Check sheet for the modelled part. Datum: model origin and axes. Units: mm. Face numbers are marked on the shaded views. A direction names the side the tool comes from. Round coordinates to 2 decimals unless told otherwise and drop trailing zeros. Write each loop counter-clockwise with the first axis right and the second up, starting at its lowest first coordinate (ties: lowest second). Pieces come first, ordered by that corner, then holes. Notation, with made-up numbers: (44, 16) -> (52, 16) arc R12 cw to (52, 38) -> close; hole circle Ø5 at (36, 15). An arc over 180 degrees is marked (long way). One line per item, written item: value. Start each with the question number.
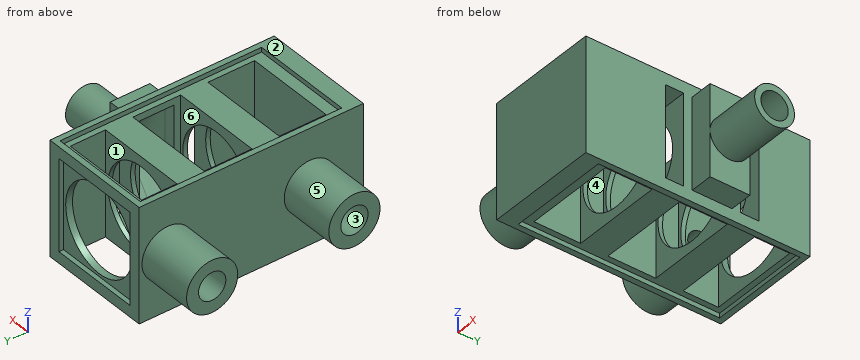
Autodesk Inventor part; units mm, degrees
ref_plane "YZ Plane" through (0, 0, 0) normal (1, 0, 0) x (0, 1, 0)
ref_plane "XZ Plane" through (0, 0, 0) normal (0, 1, 0) x (-1, 0, 0)
ref_plane "XY Plane" through (0, 0, 0) normal (0, 0, 1) x (1, 0, 0)
sketch "Sketch1" plane through (0, 0, 0) normal (0, 1, 0) x (-1, 0, 0)
  line L0 (0, 0) -> (20, 0)
  line L1 (20, 0) -> (20, 20)
  line L2 (20, 20) -> (0, 20)
  line L3 (0, 20) -> (0, 0)
  dimension "d0" = 20
  dimension "d1" = 20
extrude "Extrusion1" add sketch "Sketch1" along normal blind 34.4
sketch "Sketch2" plane through (0, 34.4, 0) normal (0, 1, 0) x (1, 0, 0)
  circle A0 centre (-10, -10) radius 7.5
  line L0 (0, 0) -> (-20, 0)
  line L1 (0, -20) -> (0, 0)
  dimension "d4" = 10
  dimension "d5" = 10
  dimension "d6" = 15
extrude "Extrusion2" cut sketch "Sketch2" against normal blind 30
sketch "Sketch3" plane through (0, 0, 20) normal (1, 0, 0) x (0, 0, -1)
  line L0 (2, 12.2) -> (18, 12.2)
  line L1 (18, 12.2) -> (18, 9)
  line L2 (18, 9) -> (2, 9)
  line L3 (2, 9) -> (2, 12.2)
  line L4 (20, 0) -> (20, 34.4)
  line L5 (0, 0) -> (20, 0)
  dimension "d9" = 3.2
  dimension "d12" = 16
  dimension "d13" = 2
  dimension "d14" = 9
extrude "Extrusion3" cut sketch "Sketch3" against normal blind 18
sketch "Sketch4" plane through (0, 0, 20) normal (1, 0, 0) x (0, 0, -1)
  line L0 (2, 25.4) -> (18, 25.4)
  line L1 (18, 25.4) -> (18, 22.2)
  line L2 (18, 22.2) -> (2, 22.2)
  line L3 (2, 22.2) -> (2, 25.4)
  line L4 (20, 0) -> (20, 34.4)
  line L5 (0, 0) -> (20, 0)
  line L6 (2, 12.2) -> (18, 12.2)
  dimension "d17" = 2
  dimension "d18" = 16
  dimension "d19" = 3.2
  dimension "d21" = 10
extrude "Extrusion4" cut sketch "Sketch4" against normal blind 18
sketch "Sketch5" plane through (0, 34.4, 0) normal (0, 1, 0) x (1, 0, 0)
  line L0 (-18, -18) -> (-2, -18)
  line L1 (-2, -18) -> (-2, -2)
  line L2 (-2, -2) -> (-18, -2)
  line L3 (-18, -2) -> (-18, -18)
  line L4 (-20, 0) -> (-20, -20)
  line L5 (-20, -20) -> (0, -20)
  line L6 (0, -20) -> (0, 0)
  line L7 (0, 0) -> (-20, 0)
  dimension "d24" = 2
  dimension "d25" = 2
  dimension "d26" = 2
  dimension "d27" = 2
extrude "Extrusion5" cut sketch "Sketch5" against normal blind 0.8 contours L3 L2 L1 L0
sketch "Sketch10" plane through (0, 0, 20) normal (1, 0, 0) x (0, 0, -1)
  line L0 (2, 20.2) -> (18, 20.2)
  line L1 (18, 20.2) -> (18, 14.2)
  line L2 (18, 14.2) -> (2, 14.2)
  line L3 (2, 14.2) -> (2, 20.2)
  line L4 (18, 22.2) -> (2, 22.2)
  line L5 (0, 0) -> (0, 34.4)
  line L6 (2, 12.2) -> (18, 12.2)
  line L7 (20, 0) -> (20, 34.4)
  dimension "d46" = 2
  dimension "d47" = 2
  dimension "d48" = 2
  dimension "d49" = 2
extrude "Extrusion7" cut sketch "Sketch10" against normal blind 17.5
sketch "Sketch6" plane through (0, 0, 20) normal (1, 0, 0) x (0, 0, -1)
  line L0 (2, 20.7) -> (18, 20.7)
  line L1 (18, 20.7) -> (18, 13.7)
  line L2 (18, 13.7) -> (2, 13.7)
  line L3 (2, 13.7) -> (2, 20.7)
  line L4 (0, 0) -> (0, 34.4)
  line L5 (20, 0) -> (20, 34.4)
  line L6 (18, 22.2) -> (2, 22.2)
  line L7 (2, 12.2) -> (18, 12.2)
  dimension "d30" = 2
  dimension "d31" = 2
  dimension "d32" = 1.5
  dimension "d33" = 1.5
extrude "Extrusion6" add sketch "Sketch6" along normal blind 4
sketch "Sketch7" plane through (4, 0, 20) normal (1, 0, 0) x (0, 0, -1)
  circle A0 centre (10, 17.2) radius 2.4
  line L0 (18, 20.7) -> (2, 20.7)
  line L1 (18, 13.7) -> (18, 20.7)
  point P0 (20, 0)
  dimension "d36" = 4.8
  dimension "d37" = 3.5
  dimension "d38" = 8
loft "Loft2" cut profiles "Sketch10", "Sketch7"
sketch "Sketch11" plane through (4, 0, 20) normal (1, 0, 0) x (0, 0, -1)
  circle A0 centre (10, 17.2) radius 3.5
  line L0 (2, 13.7) -> (18, 13.7)
  line L1 (18, 13.7) -> (18, 20.7)
  point P0 (20, 0)
  dimension "d56" = 7
  dimension "d57" = 3.5
  dimension "d58" = 8
extrude "Extrusion8" add sketch "Sketch11" along normal blind 10
sketch "Sketch12" plane through (14, 17.2, 10) normal (1, 0, 0) x (0, 0, -1)
  circle A0 centre (0, 0) radius 2.4
  circle A1 centre (0, 0) radius 3.5
  line L0 (8, -3.5) -> (8, 3.5)
  point P0 (10, -17.2)
  dimension "d62" = 4.8
  dimension "d63" = 0
  dimension "d64" = 8
extrude "Extrusion9" cut sketch "Sketch12" against normal blind 10 contours A0
sketch "Sketch13" plane through (-20, 0, 0) normal (-1, 0, 0) x (0, 0, 1)
  circle A0 centre (10, 4.4) radius 4.5
  line L0 (0, 0) -> (0, 34.4)
  line L1 (0, 0) -> (20, 0)
  dimension "d67" = 9
  dimension "d68" = 10
  dimension "d69" = 4.4
sketch "Sketch14" plane through (-20, 0, 0) normal (-1, 0, 0) x (0, 0, 1)
  circle A0 centre (10, 4.4) radius 2.4
  line L0 (20, 0) -> (20, 34.4)
  line L1 (0, 0) -> (0, 34.4)
  line L2 (0, 0) -> (20, 0)
  dimension "d71" = 10
  dimension "d72" = 4.4
  dimension "d90" = 4.8
extrude "Extrusion10" cut sketch "Sketch14" against normal blind 4
extrude "Extrusion11" add sketch "Sketch13" along normal blind 10
sketch "Sketch15" plane through (-30, 4.4, 10) normal (-1, 0, 0) x (0, 0, 1)
  circle A0 centre (0, 0) radius 2.4
  point P0 (-10, -4.4)
  dimension "d77" = 4.8
extrude "Extrusion12" cut sketch "Sketch15" against normal blind 10
sketch "Sketch16" plane through (-20, 0, 20) normal (-1, 0, 0) x (0, 0, 1)
  circle A0 centre (-10, 29.4) radius 4.5
  line L0 (0, 0) -> (0, 34.4)
  line L1 (-20, 34.4) -> (0, 34.4)
  point P0 (-20, 0)
  dimension "d80" = 10
  dimension "d81" = 5
  dimension "d82" = 9
extrude "Extrusion13" add sketch "Sketch16" along normal blind 10
sketch "Sketch17" plane through (-30, 29.4, 10) normal (-1, 0, 0) x (0, 0, 1)
  circle A0 centre (0, 0) radius 2.4
  point P0 (-10, -29.4)
  dimension "d85" = 4.8
extrude "Extrusion14" cut sketch "Sketch17" against normal blind 14
sketch "Sketch18" plane through (0, 0, 0) normal (0, -1, 0) x (1, 0, 0)
  line L0 (-20, 20) -> (0, 20)
  line L1 (0, 20) -> (0, 0)
  line L2 (-20, 20) -> (0, 20)
  line L3 (0, 20) -> (0, 0)
  line L4 (0, 0) -> (-20, 0)
  line L5 (-20, 0) -> (-20, 20)
extrude "Extrusion15" add sketch "Sketch18" along normal blind 5
sketch "Sketch19" plane through (-20, 34.4, 20) normal (0, 0, 1) x (1, 0, 0)
  line L0 (2, -26.2) -> (18, -26.2)
  line L1 (18, -26.2) -> (18, -34.4)
  line L2 (18, -34.4) -> (2, -34.4)
  line L3 (2, -34.4) -> (2, -26.2)
  line L4 (20, -39.4) -> (0, -39.4)
  line L5 (20, -39.4) -> (20, 0)
  line L6 (0, -39.4) -> (0, 0)
  point P0 (20, -34.4)
  dimension "d91" = 13.2
  dimension "d92" = 5
  dimension "d93" = 2
  dimension "d94" = 2
extrude "Extrusion16" cut sketch "Sketch19" against normal blind 20
sketch "Sketch20" plane through (-20, 34.4, 20) normal (0, 0, 1) x (1, 0, 0)
  line L0 (18, -21.4) -> (2, -21.4)
  line L1 (2, -21.4) -> (2, -13)
  line L2 (2, -13) -> (18, -13)
  line L3 (18, -13) -> (18, -21.4)
  line L4 (0, -39.4) -> (0, 0)
  line L5 (20, -39.4) -> (20, 0)
  line L6 (20, -39.4) -> (0, -39.4)
  point P0 (20, -34.4)
  dimension "d97" = 2
  dimension "d98" = 2
  dimension "d99" = 18
  dimension "d100" = 8.4
extrude "Extrusion17" cut sketch "Sketch20" against normal blind 20
sketch "Sketch21" plane through (-20, 34.4, 20) normal (0, 0, 1) x (1, 0, 0)
  line L0 (18, -8.2) -> (2, -8.2)
  line L1 (2, -8.2) -> (2, -2)
  line L2 (2, -2) -> (18, -2)
  line L3 (18, -2) -> (18, -8.2)
  line L4 (20, -39.4) -> (20, 0)
  line L5 (0, -39.4) -> (0, 0)
  line L6 (0, 0) -> (20, 0)
  point P0 (20, -34.4)
  dimension "d103" = 2
  dimension "d104" = 2
  dimension "d105" = 2
  dimension "d106" = 8.2
extrude "Extrusion18" cut sketch "Sketch21" against normal blind 20
sketch "Sketch22" plane through (-20, 34.4, 20) normal (0, 0, 1) x (1, 0, 0)
  line L0 (1, -1) -> (19, -1)
  line L1 (19, -1) -> (19, -36.4)
  line L2 (19, -36.4) -> (1, -36.4)
  line L3 (1, -36.4) -> (1, -1)
  line L4 (0, 0) -> (20, 0)
  line L5 (20, -39.4) -> (20, 0)
  line L6 (0, -39.4) -> (0, 0)
  line L7 (18, -34.4) -> (2, -34.4)
  point P0 (20, -34.4)
  dimension "d109" = 1
  dimension "d110" = 1
  dimension "d112" = 1
  dimension "d115" = 2
extrude "Extrusion19" cut sketch "Sketch22" against normal blind 0.8
sketch "Sketch23" plane through (0, 34.4, 0) normal (0, 0, -1) x (-1, 0, 0)
  line L0 (1, -36.4) -> (19, -36.4)
  line L1 (19, -36.4) -> (19, -1)
  line L2 (19, -1) -> (1, -1)
  line L3 (1, -1) -> (1, -36.4)
  line L4 (0, 0) -> (20, 0)
  line L5 (0, 0) -> (0, -39.4)
  line L6 (20, -39.4) -> (20, 0)
  line L7 (18, -34.4) -> (2, -34.4)
  point P0 (0, -34.4)
  dimension "d116" = 1
  dimension "d117" = 1
  dimension "d118" = 1
  dimension "d119" = 2
extrude "Extrusion20" cut sketch "Sketch23" against normal blind 0.8
properties part number "HDAcell_Daniela_thickelecrode_08172020"
1. Cross-section at B-B (z = 18.5). Record the cut outline in (x, y), plus the area to 3 significant figures.
2. Cross-section at A-A (y = 4.4). Record the cut outline in (x, z), plus the area to 3 significant figures.
3. Depth check by flat-ended pin: pin 1 Ø5 at (x, z) = (-6, 12) entering from +Y; pin 2 Ø3.5 at (x, y) = (-10, 23) entering from +Z; pin 3 Ø1.5 at (y, z) = (0.5, 12) entering from +X. Enter the tip coordinate at first touch or a pass-through.
4. Cross-section at C-C (x = -27). Record the cut outline in (y, z), plus the area to 3 significant figures.
5. Access from +Z, -Z, +X, -X, +Y, -Y to the whole of each face (thin tool, end or side, straight path). Record for the marked faces 4, 5 and 6.
6. Material ranges on probe 1 along Y at (x, z) = (-23, 10); probe 2 along Y at (x, z) = (-7, 18.5); probe 3 along Z at (x, y) = (-15.5, 10.5), recorded low to high.
7. Cross-section at D-D (x = -10). Give the number of separate pieces and of enclosed holes in the cut face, plus the area to 3 significant figures.
8. Release check for a two-part mould opening along Z. For the marked faces 1, 2 and 3 record: +Z half, -Z half, draft (parallel to the pull), parting line (faces both ways), or undercut.
Working result:
1. outline: (-20, -5) -> (0, -5) -> (0, 34.4) -> (-20, 34.4) -> close; hole (-18, 0) -> (-2, 0) -> (-2, 8.2) -> (-18, 8.2) -> close; hole (-18, 13) -> (-2, 13) -> (-2, 21.4) -> (-18, 21.4) -> close; hole (-18, 26.2) -> (-2, 26.2) -> (-2, 32.4) -> (-18, 32.4) -> close
1. area: 423 mm^2
2. outline: (-30, 5.5) -> (-20, 5.5) -> (-20, 0) -> (-19, 0) -> (-19, 0.8) -> (-18, 0.8) -> (-18, 7.6) -> (-30, 7.6) -> close; (-30, 12.4) -> (-18, 12.4) -> (-18, 19.2) -> (-19, 19.2) -> (-19, 20) -> (-20, 20) -> (-20, 14.5) -> (-30, 14.5) -> close; (-2, 0.8) -> (-1, 0.8) -> (-1, 0) -> (0, 0) -> (0, 20) -> (-1, 20) -> (-1, 19.2) -> (-2, 19.2) -> close
2. area: 109 mm^2
3. pin 1: stops at y = 0
3. pin 2: stops at z = 19.2
3. pin 3: stops at x = 0
4. outline: circle Ø9 at (4.4, 10); circle Ø9 at (29.4, 10); hole circle Ø4.8 at (4.4, 10); hole circle Ø4.8 at (29.4, 10)
4. area: 91.0 mm^2
5. face 4: +X
5. face 5: -X
5. face 6: +Z, -Z
6. probe 1: y = -0.1 to 2, 6.8 to 8.9, 24.9 to 27, 31.8 to 33.9
6. probe 2: y = -5 to 0, 8.2 to 13, 21.4 to 26.2, 32.4 to 34.4
6. probe 3: z = 0.8 to 2, 18 to 19.2
7. separate pieces: 7
7. enclosed holes: 0
7. area: 131 mm^2
8. face 1: draft
8. face 2: +Z half
8. face 3: undercut
